```python
from build123d import *

# Parameters (mm, degrees)
SKETCH1_W           = 56
SKETCH1_H           = 20
BOSS_EXTRUDE1_DEPTH = 2
SKETCH2_W           = 2
SKETCH2_H           = 20
BOSS_EXTRUDE2_DEPTH = 35
SKETCH3_R           = 4
SKETCH3_R_2         = 1.5
CUT_EXTRUDE1_DEPTH  = 70.744065851
SKETCH4_R           = 1.5
SKETCH4_R_2         = 3
CUT_EXTRUDE2_DEPTH  = 67.983988806


with BuildPart() as part:
    # Sketch1 → Boss-Extrude1 (new body)
    with BuildSketch(Plane(origin=(0, 0, 0), x_dir=(1, 0, 0), z_dir=(0, 1, 0))):
        with Locations((25.875968992, 8.953488372)):
            Rectangle(SKETCH1_W, SKETCH1_H)
    extrude(amount=BOSS_EXTRUDE1_DEPTH)

    # Sketch2 → Boss-Extrude2 (add)
    with BuildSketch(Plane(origin=(0, 2, 0), x_dir=(1, 0, 0), z_dir=(0, 1, 0))):
        with Locations((-1.124031008, 8.953488372)):
            Rectangle(SKETCH2_W, SKETCH2_H)
        with Locations((52.875968992, 8.953488372)):
            Rectangle(SKETCH2_W, SKETCH2_H)
    extrude(amount=BOSS_EXTRUDE2_DEPTH)

    # Sketch3 → Cut-Extrude1 (cut, through all)
    with BuildSketch(Plane.ZY.offset(2.124031008)):
        with Locations((-8.953488372, 27)):
            Circle(SKETCH3_R)
        with Locations((-15.953488372, 27)):
            Circle(SKETCH3_R_2)
        with Locations((-1.953488372, 27)):
            Circle(SKETCH3_R_2)
        with Locations((-8.953488372, 34)):
            Circle(SKETCH3_R_2)
        with Locations((-8.953488372, 20)):
            Circle(SKETCH3_R_2)
    extrude(amount=-CUT_EXTRUDE1_DEPTH, mode=Mode.SUBTRACT)

    # Sketch4 → Cut-Extrude2 (cut, through all)
    with BuildSketch(Plane(origin=(0, 2, 0), x_dir=(1, 0, 0), z_dir=(0, 1, 0))):
        with Locations(Location((30.825468992, 4.003988372, 0), (0, 0, 270))):
            Circle(SKETCH4_R)
        with Locations(Location((20.926468992, 4.003988372, 0), (0, 0, 270))):
            Circle(SKETCH4_R)
        with Locations(Location((30.825468992, 13.902988372, 0), (0, 0, 270))):
            Circle(SKETCH4_R)
        with Locations(Location((20.926468992, 13.902988372, 0), (0, 0, 270))):
            Circle(SKETCH4_R)
        with Locations(Location((25.875968992, 8.953488372, 0), (0, 0, 270))):
            Circle(SKETCH4_R_2)
        with Locations(Location((40.724468992, 4.003988372, 0), (0, 0, 270))):
            Circle(SKETCH4_R)
        with Locations(Location((40.724468992, 13.902988372, 0), (0, 0, 270))):
            Circle(SKETCH4_R)
        with Locations(Location((11.027468992, 13.902988372, 0), (0, 0, 270))):
            Circle(SKETCH4_R)
        with Locations(Location((11.027468992, 4.003988372, 0), (0, 0, 270))):
            Circle(SKETCH4_R)
    extrude(amount=-CUT_EXTRUDE2_DEPTH, mode=Mode.SUBTRACT)


solid = part.part
```
Check sheet for the modelled part. Datum: model origin and axes. Units: mm. A direction names the side the tool comes from. Round coordinates to 2 decimals unless told otherwise and drop trailing zeros. Write each loop counter-clockwise with the first axis right and the second up, starting at its lowest first coordinate (ties: lowest second). Pieces come first, ordered by that corner, then holes. Notation, with made-up numbers: (73.25, 27) -> (115.25, 27) arc R21 cw to (115.25, 38) -> close; hole circle Ø6 at (35, 4). An arc over 180 degrees is marked (long way). Put each result on its own line as item: value.
(1) Go/stop test with flat-tipped pins: pin 1 Ø9 at (y, z) = (27, -8.95) entering from +X; pin 2 Ø10 at (x, z) = (13.5, -16) entering from +Y. Record where each tip stops, or that it passes through.
Values found:
pin 1: stops at x = 53.88
pin 2: stops at y = 2
(2) Sectioned sample at A-A (y = 27). Count the separate pieces of the cut face and the enclosed holes in it, plus the area to 3 significant figures.
Values found:
separate pieces: 8
enclosed holes: 0
area: 24.0 mm^2
(3) Sectioned sample at B-B (y = 20). Enter the section's corners in (x, z).
Values found:
outline: (-2.12, -18.95) -> (-0.12, -18.95) -> (-0.12, -10.45) -> (-2.12, -10.45) -> close; (-2.12, -7.45) -> (-0.12, -7.45) -> (-0.12, 1.05) -> (-2.12, 1.05) -> close; (51.88, -18.95) -> (53.88, -18.95) -> (53.88, -10.45) -> (51.88, -10.45) -> close; (51.88, -7.45) -> (53.88, -7.45) -> (53.88, 1.05) -> (51.88, 1.05) -> close
(4) Sectioned sample at C-C (x = 27.5). Enter the section's corners in (y, z), plus the area to 3 significant figures.
Values found:
outline: (0, -18.95) -> (2, -18.95) -> (2, -11.48) -> (0, -11.48) -> close; (0, -6.43) -> (2, -6.43) -> (2, 1.05) -> (0, 1.05) -> close
area: 29.9 mm^2
(5) Tool access check on faces 4 (the face through (26, 1, -18.953)), 5 (the face through (26, 2, -5)). Record the directions out of +Z, -Z, +X, -X, +Y, -Y that give a thin tool (end or side, any length) a straight path to the whole face; none if there is none.
Values found:
face 4: -Z, +X, -X, +Y, -Y
face 5: +Z, -Z, +Y
(6) Material ranges on line 1 (X direction, y = 7, z = -6.75); line 2 (Y direction, x = 36, z = -6.25), recorded low to high.
Values found:
line 1: x = -2.12 to -0.12, 51.88 to 53.88
line 2: y = 0 to 2
(7) Sectioned sample at D-D (z = -1.5). Enter the section's corners in (x, y), plus the area to 3 significant figures.
Values found:
outline: (-2.12, 0) -> (53.88, 0) -> (53.88, 25.57) -> (51.88, 25.57) -> (51.88, 2) -> (-0.12, 2) -> (-0.12, 25.57) -> (-2.12, 25.57) -> close; (-2.12, 28.43) -> (-0.12, 28.43) -> (-0.12, 37) -> (-2.12, 37) -> close; (51.88, 28.43) -> (53.88, 28.43) -> (53.88, 37) -> (51.88, 37) -> close
area: 241 mm^2
(8) Mould release check, pull along X, two halves, no side actions. Record for faces 1 (the face through (-1.138, 33.087, -10.144)), 2 (the face through (-2.124, 18, -9)), 3 (the face through (32.313, 1.014, -14.098)): released by +X, released by -X, zero draft, split by the parting line, or undercut.
Values found:
face 1: zero draft
face 2: released by -X
face 3: undercut
